Part print with two shaded views. Sizes in mm from the minimum x, y, z corner. A direction names the side the tool comes from. Coordinates: 2 decimals unless noted, no trailing zeros. Loops run counter-clockwise (first coordinate to the right, second up) from the corner with the lowest first, then second, coordinate; pieces in that order, holes last. Notation, with made-up numbers: (13.25, 55.5) -> (23.25, 55.5) arc R15 ccw to (23.25, 64.5) -> close; hole circle Ø5 at (5.5, 16.5). An arc over 180 degrees is marked (long way). Use one line per item in the form item = value.
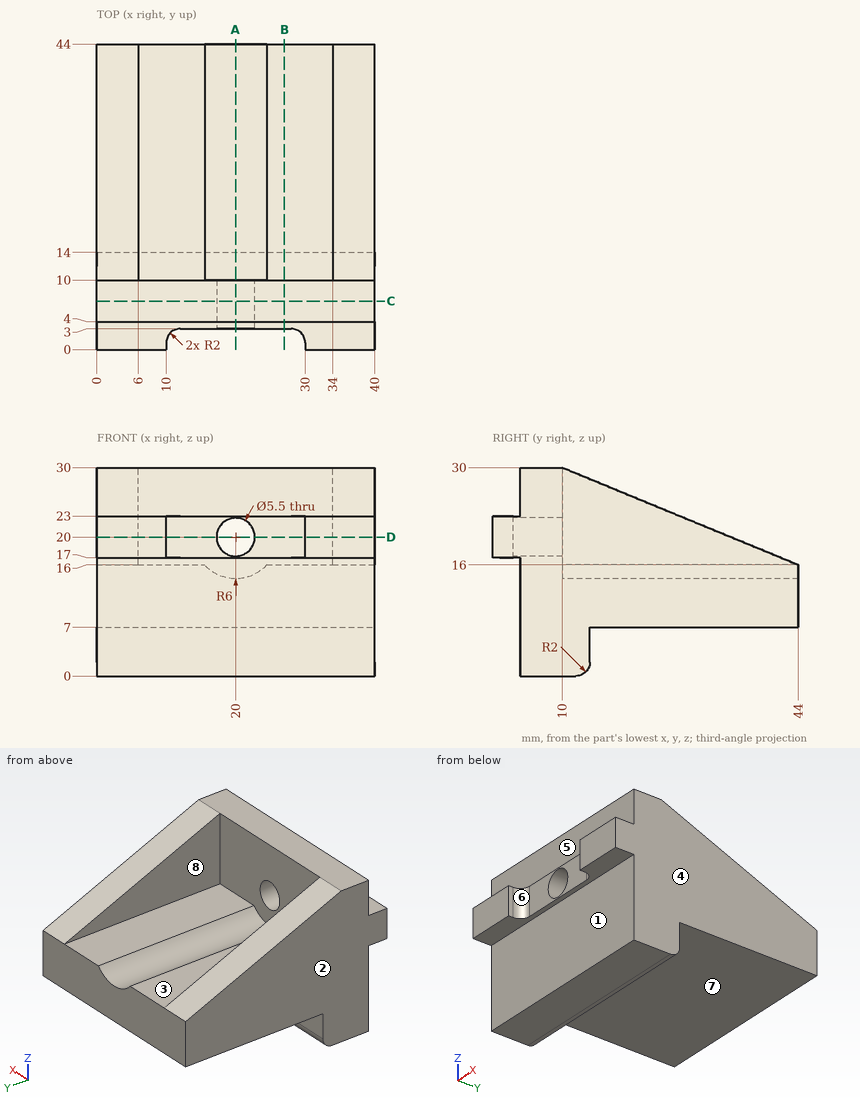
Q1. Band-saw the part on D-D, the plane z = 20. Write the cut outline in (x, y), and give its area (3 significant figures).
Result:
outline = (0, 0) -> (10, 0) -> (10, 1) arc R2 cw to (12, 3) -> (17.25, 3) -> (17.25, 10) -> (6, 10) -> (6, 34.29) -> (0, 34.29) -> close; (22.75, 3) -> (28, 3) arc R2 cw to (30, 1) -> (30, 0) -> (40, 0) -> (40, 34.29) -> (34, 34.29) -> (34, 10) -> (22.75, 10) -> close
area = 595 mm2
Q2. Band-saw the part on A-A, the plane x = 20. Write the cut outline in (y, z), and give its area (3 significant figures).
Result:
outline = (3, 17) -> (4, 17) -> (4, 0) -> (12, 0) arc R2 ccw to (14, 2) -> (14, 7) -> (44, 7) -> (44, 14) -> (10, 14) -> (10, 17.25) -> (3, 17.25) -> close; (3, 22.75) -> (10, 22.75) -> (10, 30) -> (4, 30) -> (4, 23) -> (3, 23) -> close
area = 413 mm2
Q3. Band-saw the part on C-C, the plane y = 7. Write the cut outline in (x, z), and give its area (3 significant figures).
Result:
outline = (0, 0) -> (40, 0) -> (40, 30) -> (0, 30) -> close; hole circle Ø5.5 at (20, 20)
area = 1,180 mm2
Q4. Band-saw the part on B-B, the plane x = 27. Write the cut outline in (y, z).
Result:
outline = (3, 17) -> (4, 17) -> (4, 0) -> (12, 0) arc R2 ccw to (14, 2) -> (14, 7) -> (44, 7) -> (44, 16) -> (10, 16) -> (10, 30) -> (4, 30) -> (4, 23) -> (3, 23) -> close
Q5. Pin check, flat tips, straight feed: pin 1 Ø6.5 at (x, z) = (16.5, 19.5) entering from -Y; pin 2 Ø1.2 at (x, y) = (22, 2.5) entering from +Z; pin 3 Ø5 at (x, z) = (27.5, 3) entering from -Y. Stop position of each tip, or through.
Result:
pin_1 = 3
pin_2 = 23
pin_3 = 4
Q6. Mould opens along X. For the marked faces 1, 2, 3 and 4 say: released by +X, released by -X, zero draft, split by the parting line, or undercut.
Result:
face_1 = zero draft
face_2 = released by -X
face_3 = undercut
face_4 = released by +X
Q7. Which spindle directions (+Z, -Z, +X, -X, +Y, -Y) get a long thin tool onto all of the face, cutting with end or side? Do the marked faces 5, 6, 7 and 8. Say none if no direction does.
Result:
face_5 = +Z, +X, -X, -Y
face_6 = +Z, -Z, -Y
face_7 = -Z, +X, -X, +Y
face_8 = +Z, +Y
Q8. Wall check: line 1 along Z through (x, y) = (20, 5); line 2 along X through (y, z) = (17, 20.25); line 3 along Y through (x, z) = (15.5, 17.25). Give the ranges that are in metal, low to high.
Result:
line_1 = 0 to 17.25, 22.75 to 30
line_2 = 0 to 6, 34 to 40
line_3 = 3 to 10
